Source: CAD feature listing. Evaluate the final solid. Frame: model axes, mm. A direction names the side the tool comes from. Coordinates: 2 decimals unless noted, no trailing zeros. Write each loop counter-clockwise with the first axis right and the second up, starting at its lowest first coordinate (ties: lowest second). Pieces come first, ordered by that corner, then holes. Notation, with made-up numbers: (11, -20) -> (47, -20) arc R30 cw to (47, 8) -> close; hole circle Ø6 at (43, 20.5). An arc over 180 degrees is marked (long way). One line per item, written item: value. Start each with the question number.
1. Access query for faces 1 (the flat face through (-16, -47, 63.5)), 2 (the flat face through (0, -18.9, 48.5)). Directions: +Z, -Z, +X, -X, +Y, -Y. A direction counts if a zero-diameter tool reaches every point of the face in a straight line with its end or side. Return the directions, or none.
2. Line query: line 1 (Z direction, x = -31, y = -8); line 2 (Y direction, x = -31.75, z = 71); line 3 (X direction, y = -63, z = 52). Output: solid intervals per line, ascending.
3. Section query A-A, the plane x = -31.75. Output: boundary loops of the cut face in (y, z), and give its area (3 significant figures).
4. Mould query, pull axis X, two halves, no side actions, for faces 3 (the cylindrical face through (-34.5, -33.83, 69.76)), 4 (the flat face through (-46, -19.05, 32)), 5 (the flat face through (-76.2, -29, 39)). Classes: released by +X, released by -X, zero draft, split by the parting line, or undercut.
5. First-contact query: P1, Ø5, axis at y = -68.5, z = 19, coming from the +X side; P2, Ø1, axis at x = -12, z = 26.5, coming from the -Y side. Flat tips, straight axial feed; report the tip coordinate or a pass-through.
6. Section query C-C, the plane y = -30.5. Output: boundary loops of the cut face in (x, z), and give its area (3 significant figures).
7. Section query B-B, the plane z = 31.75. Output: boundary loops of the cut face in (x, y), and give its area (3 significant figures).
8. Section query D-D, the plane x = -65.5. Output: boundary loops of the cut face in (y, z), and give its area (3 significant figures).
from build123d import *

# Parameters (mm, degrees)
F0_W      = 76.2
F0_H      = 76.2
F1_DEPTH  = 19.05
F3_DEPTH  = 57.15
F4_R      = 12.7
F5_DEPTH  = 12.7
F6_R      = 12.7
F7_DEPTH  = 19.05
F8_R      = 6.35
F9_SIZE   = 6.35
F10_R     = 12.7
F11_DEPTH = 12.7


with BuildPart() as f1:
    # F0 (on Front) → F1 (new body)
    with BuildSketch(Plane.XZ):
        with Locations((-38.1, 38.1)):
            Rectangle(F0_W, F0_H)
    extrude(amount=F1_DEPTH)

    # F2 (on face) → F3 (join)
    with BuildSketch(Plane.XZ.offset(19.05)):
        Polygon((-76.2, 76.2), (-76.2, 0), (-63.5, 0), (-63.5, 63.5), (0, 63.5), (0, 76.2), align=None)
    extrude(amount=F3_DEPTH)

    # F4 (on face) → F5 (cut)
    with BuildSketch(Plane(origin=(0, 0, 63.5), x_dir=(1, 0, 0), z_dir=(0, 0, -1))):
        with Locations((-31.75, 46.228)):
            Circle(F4_R)
    extrude(amount=-F5_DEPTH, mode=Mode.SUBTRACT)

    # F6 (on face) → F7 (cut)
    with BuildSketch(Plane.XZ.offset(19.05)):
        with Locations((-31.75, 31.75)):
            Circle(F6_R)
    extrude(amount=-F7_DEPTH, mode=Mode.SUBTRACT)

    # F8
    f8_edges = [f1.edges().sort_by_distance(p)[0] for p in [
        (-63.5, -47.625, 63.5),
    ]]
    fillet(f8_edges, radius=F8_R)

    # F9
    f9_edges = [f1.edges().sort_by_distance(p)[0] for p in [
        (0, -9.525, 0),
        (-69.85, -76.2, 0),
        (0, -76.2, 69.85),
    ]]
    chamfer(f9_edges, length=F9_SIZE)

    # F10 (on face) → F11 (cut)
    with BuildSketch(Plane.YZ.offset(-63.5)):
        with Locations((-46.228, 31.75)):
            Circle(F10_R)
    extrude(amount=-F11_DEPTH, mode=Mode.SUBTRACT)


solid = f1.part
Computed values:
1. face 1: -Z, +X, -Y
1. face 2: +Z, -Z, +X, +Y, -Y
2. line 1: z = 0 to 19.07, 44.43 to 76.2
2. line 2: y = -76.2 to -58.93, -33.53 to 0
2. line 3: x = -76.2 to -63.5
3. outline: (-76.2, 63.5) -> (-58.93, 63.5) -> (-58.93, 76.2) -> (-76.2, 76.2) -> close; (-33.53, 63.5) -> (-19.05, 63.5) -> (-19.05, 44.45) -> (0, 44.45) -> (0, 76.2) -> (-33.53, 76.2) -> close; (-19.05, 0) -> (0, 0) -> (0, 19.05) -> (-19.05, 19.05) -> close
3. area: 1,370 mm²
4. face 3: undercut
4. face 4: zero draft
4. face 5: released by -X
5. P1: stops at x = -63.5
5. P2: stops at y = -19.05
6. outline: (-76.2, 0) -> (-63.5, 0) -> (-63.5, 57.15) arc R6.35 cw to (-57.15, 63.5) -> (0, 63.5) -> (0, 76.2) -> (-76.2, 76.2) -> close
6. area: 1,780 mm²
7. outline: (-76.2, -76.2) -> (-63.5, -76.2) -> (-63.5, -58.93) -> (-76.2, -58.93) -> close; (-76.2, -33.53) -> (-63.5, -33.53) -> (-63.5, -19.05) -> (-44.45, -19.05) -> (-44.45, 0) -> (-76.2, 0) -> close; (-19.05, -19.05) -> (0, -19.05) -> (0, 0) -> (-19.05, 0) -> close
7. area: 1,370 mm²
8. outline: (-76.2, 6.35) -> (-69.85, 0) -> (0, 0) -> (0, 76.2) -> (-76.2, 76.2) -> close; hole circle Ø25.4 at (-46.23, 31.75)
8. area: 5,280 mm²
